Can you work these out from the model? Positions are in its coordinate system, mm. Give positions to 0.01 mm unless a question says otherwise; leave off trailing zeros. Order: outer loops, then holes, each group sorted by start corner. A loop starts at its lowest first (then second) coordinate and runs counter-clockwise, first axis right, second up. Notation, with made-up numbers: (61.25, 31.25) - (89.25, 31.25) arc R26 ccw to (89.25, 67.25) - close; hole circle Ø4 at (86, -10.75). An arc over 180 degrees is marked (long way). Return JSON: item names as keys, results as strings.
```python
from build123d import *

# Parameters (mm, degrees)
BOSS_EXTRUDE1_DEPTH = 3.175
FILLET1_R           = 5.08
SKETCH2_R           = 2.413
CUT_EXTRUDE1_DEPTH  = 14.153467


with BuildPart() as part:
    # Sketch1 → Boss-Extrude1 (new body)
    with BuildSketch(Plane(origin=(0, 0, 0), x_dir=(1, 0, 0), z_dir=(0, 1, 0))):
        Polygon((0, 0), (393.7, 0), (196.85, 340.95420147), align=None)
    extrude(amount=BOSS_EXTRUDE1_DEPTH)

    # Fillet1
    fillet1_edges = [part.edges().sort_by_distance(p)[0] for p in [
        (196.85, 1.5875, -340.95420147),
        (393.7, 1.5875, 0),
        (0, 1.5875, 0),
    ]]
    fillet(fillet1_edges, radius=FILLET1_R)

    # Sketch2 → Cut-Extrude1 (cut)
    with BuildSketch(Plane(origin=(0, 3.175, 0), x_dir=(1, 0, 0), z_dir=(0, 1, 0))):
        with Locations((37.394976935, 21.59)):
            Circle(SKETCH2_R)
        with Locations((59.392022192, 34.29)):
            Circle(SKETCH2_R)
        with Locations((70.39054482, 40.64)):
            Circle(SKETCH2_R)
        with Locations((114.384635332, 66.04)):
            Circle(SKETCH2_R)
        with Locations((103.386112704, 59.69)):
            Circle(SKETCH2_R)
        with Locations((196.85, 297.77420147)):
            Circle(SKETCH2_R)
        with Locations((196.85, 272.37420147)):
            Circle(SKETCH2_R)
        with Locations((196.85, 259.67420147)):
            Circle(SKETCH2_R)
        with Locations((196.85, 221.57420147)):
            Circle(SKETCH2_R)
        with Locations((196.85, 208.87420147)):
            Circle(SKETCH2_R)
        with Locations((279.315364668, 66.04)):
            Circle(SKETCH2_R)
        with Locations((290.313887296, 59.69)):
            Circle(SKETCH2_R)
        with Locations((323.30945518, 40.64)):
            Circle(SKETCH2_R)
        with Locations((334.307977808, 34.29)):
            Circle(SKETCH2_R)
        with Locations((356.305023065, 21.59)):
            Circle(SKETCH2_R)
    extrude(amount=-CUT_EXTRUDE1_DEPTH, mode=Mode.SUBTRACT)


solid = part.part
```
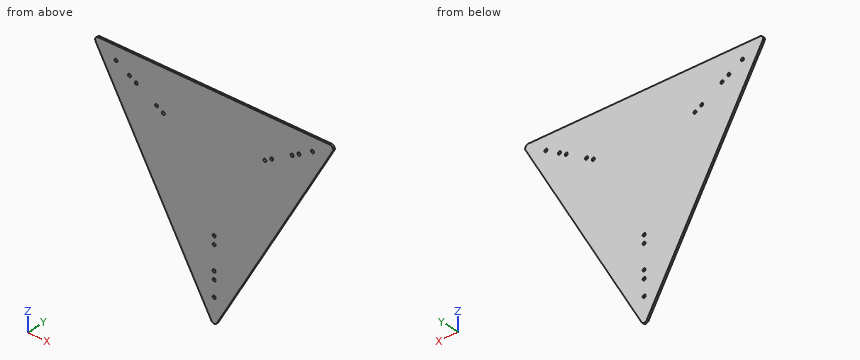
1. If I drill on L1, parallel to Z at x = 196.85, y = 1.65; L2, parallel to X at y = 2.3, z = -59.69; L3, parallel to X at y = 1.2, z = -40.64, over which ranges is the centre line in solid material (lowest first)? Write a range as [from, to].
Checks:
{"L1": "[-335.87, -300.19], [-295.36, -274.79], [-269.96, -262.09], [-257.26, -223.99], [-219.16, -211.29], [-206.46, 0]", "L2": "[34.46, 100.97], [105.8, 287.9], [292.73, 359.24]", "L3": "[23.46, 67.98], [72.8, 320.9], [325.72, 370.24]"}
2. Suppose I cut it at B-B (x = 92.5). List the corners of the cut face in (y, z) for me (3 decimals), plus the area to 3 significant figures.
Checks:
{"outline": "(0, -160.215) - (3.175, -160.215) - (3.175, 0) - (0, 0) - close", "area": "509 mm^2"}
3. Suppose I cut it at C-C (z = -49). List the corners of the cut face in (x, y) for me (3 decimals), plus the area to 3 significant figures.
Checks:
{"outline": "(28.29, 0) - (365.41, 0) - (365.41, 3.175) - (28.29, 3.175) - close", "area": "1,070 mm^2"}
4. For pin 1 Ø3 at (x, z) = (70.39, -40.64) entering from +Y; pin 2 Ø7.5 at (x, z) = (37.39, -21.59) entering from -Y, each with a flat end and sliding along its axis, tell me the tip position at first contact or that it passes through.
Checks:
{"pin 1": "through", "pin 2": "y = 0"}
5. Suppose I cut it at A-A (y = 1.1). State how many separate pieces and enclosed holes the cut face has, plus the area to 3 significant figures.
Checks:
{"separate pieces": "1", "enclosed holes": "15", "area": "66,800 mm^2"}
